from build123d import *

# Parameters (mm, degrees)
SKETCH_1_R      = 2.5
EXTRUDE_1_DEPTH = 6


with BuildPart() as part:
    # Эскиз1 → Бобышка-Вытянуть1 (new body)
    with BuildSketch(Plane.XY):
        Polygon((-28, -26), (-27.75, -20), (27.75, -20), (28, -26), (38, -26), (38.25, -20), (43.45, -20), (55.95, -20), (55.95, -13.2), (54.75, -13.2), (54.75, -11), (55.95, -11), (55.95, -9.5), (59.05, -9.5), (59.05, -11), (60.25, -11), (60.25, -13.2), (59.05, -13.2), (59.05, -20), (64.25, -20), (76.75, -20), (77, -26), (87, -26), (87.25, -20), (120.5, -20), (120.5, -15.55), (115.7, -15.55), (115.7, -16.75), (113.5, -16.75), (113.5, -15.55), (112, -15.55), (112, -12.45), (113.5, -12.45), (113.5, -11.25), (115.7, -11.25), (115.7, -12.45), (120.5, -12.45), (120.5, -7.5), (132.5, -7.5), (132.5, 7.5), (120.5, 7.5), (120.5, 12.45), (115.7, 12.45), (115.7, 11.25), (113.5, 11.25), (113.5, 12.45), (112, 12.45), (112, 15.55), (113.5, 15.55), (113.5, 16.75), (115.7, 16.75), (115.7, 15.55), (120.5, 15.55), (120.5, 20), (87.25, 20), (87, 26), (77, 26), (76.75, 20), (64.25, 20), (59.05, 20), (59.05, 13.2), (60.25, 13.2), (60.25, 11), (59.05, 11), (59.05, 9.5), (55.95, 9.5), (55.95, 11), (54.75, 11), (54.75, 13.2), (55.95, 13.2), (55.95, 20), (43.45, 20), (38.25, 20), (38, 26), (28, 26), (27.75, 20), (-27.75, 20), (-28, 26), (-38, 26), (-38.25, 20), (-43.45, 20), (-55.95, 20), (-55.95, 13.2), (-54.75, 13.2), (-54.75, 11), (-55.95, 11), (-55.95, 9.5), (-59.05, 9.5), (-59.05, 11), (-60.25, 11), (-60.25, 13.2), (-59.05, 13.2), (-59.05, 20), (-71.55, 20), (-76.75, 20), (-77, 26), (-87, 26), (-87.25, 20), (-120.5, 20), (-120.5, 15.55), (-115.7, 15.55), (-115.7, 16.75), (-113.5, 16.75), (-113.5, 15.55), (-112, 15.55), (-112, 12.45), (-113.5, 12.45), (-113.5, 11.25), (-115.7, 11.25), (-115.7, 12.45), (-120.5, 12.45), (-120.5, 7.5), (-132.5, 7.5), (-132.5, -7.5), (-120.5, -7.5), (-120.5, -12.45), (-115.7, -12.45), (-115.7, -11.25), (-113.5, -11.25), (-113.5, -12.45), (-112, -12.45), (-112, -15.55), (-113.5, -15.55), (-113.5, -16.75), (-115.7, -16.75), (-115.7, -15.55), (-120.5, -15.55), (-120.5, -20), (-87.25, -20), (-87, -26), (-77, -26), (-76.75, -20), (-71.55, -20), (-59.05, -20), (-59.05, -13.2), (-60.25, -13.2), (-60.25, -11), (-59.05, -11), (-59.05, -9.5), (-55.95, -9.5), (-55.95, -11), (-54.75, -11), (-54.75, -13.2), (-55.95, -13.2), (-55.95, -20), (-43.45, -20), (-38.25, -20), (-38, -26), align=None)
        with Locations((0, 10)):
            Circle(SKETCH_1_R, mode=Mode.SUBTRACT)
    extrude(amount=EXTRUDE_1_DEPTH)


solid = part.part
Geometry: final body of the model. Coordinates: model frame, mm. A direction names the side the tool comes from. Round coordinates to 2 decimals unless told otherwise and drop trailing zeros. Loops run counter-clockwise (first coordinate to the right, second up) from the corner with the lowest first, then second, coordinate; pieces in that order, holes last. Notation, with made-up numbers: M 70,-32.5 L 122,-32.5 A23 cw 122,-2.5 Z; hole C -26,49 d9. An arc over 180 degrees is marked long. Put each result on its own line as item: value. Start each with the question number.
(1) Section query A-A (x = 0). Return loops of the section in (y, z).
(2) Contact query for flat-ended pins moving along their axis: pin 1 Ø3.5 at (x, z) = (58, 4.5) entering from -Y; pin 2 Ø1 at (x, z) = (-102.5, 1) entering from +Y; pin 3 Ø0.9 at (x, z) = (-57.5, 3) entering from +Y. Output: stop coordinate, or through.
(3) Material intervals for line 1 along Y through (x, z) = (-114.5, 5.55); line 2 along Y through (x, z) = (0, 3.05); line 3 along X through (y, z) = (-22.5, 4.6), sorted ascending. Write a range as [from, to].
(4) Draft query along Y for faces 4 (the face through (120.5, -18, 3)), 5 (the face through (-118, -12.45, 3)), 6 (the face through (-47, -20, 3)). Return one class per face: +Y half, -Y half, draft (parallel to the pull), parting line (faces both ways), or undercut.
(5) Set-up query: faces 1 (the face through (68, -20, 3)), 2 (the face through (-127, -7.5, 3)), 3 (the face through (-104, 20, 3)). Return all of +Z, -Z, +X, -X, +Y, -Y with unobstructed straight access to the full face (end or side cutting, diameter ignored); none if empty.
Findings below:
1. outline: M -20,0 L 7.5,0 L 7.5,6 L -20,6 Z; M 12.5,0 L 20,0 L 20,6 L 12.5,6 Z
2. pin 1: stops at y = -20
2. pin 2: stops at y = 20
2. pin 3: stops at y = 9.5
3. line 1: y = [-20, -16.75], [-11.25, 11.25], [16.75, 20]
3. line 2: y = [-20, 7.5], [12.5, 20]
3. line 3: x = [-87.15, -76.85], [-38.15, -27.85], [27.85, 38.15], [76.85, 87.15]
4. face 4: draft
4. face 5: undercut
4. face 6: -Y half
5. face 1: +Z, -Z, -Y
5. face 2: +Z, -Z, -X, -Y
5. face 3: +Z, -Z, -X, +Y
